from build123d import *

# Parameters (mm, degrees)
BOSS_EXTRUDE1_DEPTH                                 = 6.35
SKETCH2_W                                           = 6.35
SKETCH2_H                                           = 6.35
CUT_EXTRUDE1_DEPTH                                  = 7.35
F_8_0_199_DIAMETER_HOLE1_D                          = 5.0546
SKETCH5_W                                           = 6.35
SKETCH5_H                                           = 3.81
CUT_EXTRUDE2_DEPTH                                  = 7.35
CBORE_FOR_8_BINDING_HEAD_MACHINE_SCREW1_D           = 4.4958
CBORE_FOR_8_BINDING_HEAD_MACHINE_SCREW1_CBORE_D     = 9.525
CBORE_FOR_8_BINDING_HEAD_MACHINE_SCREW1_CBORE_DEPTH = 3.175


with BuildPart() as part:
    # Sketch1 → Boss-Extrude1 (new body)
    with BuildSketch(Plane(origin=(0, 0, 0), x_dir=(1, 0, 0), z_dir=(0, 1, 0))):
        Polygon((8.763, -10.331391255), (8.763, -15.411391255), (-1.905, -15.411391255), (-1.905, 7.448608745), (0, 7.448608745), (0, 192.868608745), (31.75, 192.868608745), (31.75, -10.331391255), align=None)
    extrude(amount=BOSS_EXTRUDE1_DEPTH)

    # Sketch2 → Cut-Extrude1 (cut, through all)
    with BuildSketch(Plane(origin=(0, 6.35, 0), x_dir=(1, 0, 0), z_dir=(0, 1, 0))):
        with Locations((3.175, 52.025608745)):
            Rectangle(SKETCH2_W, SKETCH2_H)
        with Locations((3.175, 100.285608745)):
            Rectangle(SKETCH2_W, SKETCH2_H)
        with Locations((3.175, 148.545608745)):
            Rectangle(SKETCH2_W, SKETCH2_H)
    extrude(amount=-CUT_EXTRUDE1_DEPTH, mode=Mode.SUBTRACT)

    # #8 (0.199) Diameter Hole1 (through all)
    with Locations(Plane(origin=(0, 6.35, 0), x_dir=(1, 0, 0), z_dir=(0, 1, 0))):
        with Locations((3.937, 2.368608745), (3.937, -10.331391255)):
            Hole(F_8_0_199_DIAMETER_HOLE1_D / 2)

    # Sketch5 → Cut-Extrude2 (cut, through all)
    with BuildSketch(Plane(origin=(0, 6.35, 0), x_dir=(1, 0, 0), z_dir=(0, 1, 0))):
        with Locations((3.175, -3.854391255)):
            Rectangle(SKETCH5_W, SKETCH5_H)
    extrude(amount=-CUT_EXTRUDE2_DEPTH, mode=Mode.SUBTRACT)

    # CBORE for #8 Binding Head Machine Screw1 (through all)
    with Locations(Plane(origin=(0, 6.35, 0), x_dir=(1, 0, 0), z_dir=(0, 1, 0))):
        with Locations((19.05, 173.818608745), (19.05, 142.068608745), (19.05, 15.068608745)):
            CounterBoreHole(CBORE_FOR_8_BINDING_HEAD_MACHINE_SCREW1_D / 2, CBORE_FOR_8_BINDING_HEAD_MACHINE_SCREW1_CBORE_D / 2, CBORE_FOR_8_BINDING_HEAD_MACHINE_SCREW1_CBORE_DEPTH)


solid = part.part
Read the model definition and answer for the solid it produces. Units are mm, in the model's axes. A direction names the side the tool comes from. Give positions to 0.01 mm unless a question says otherwise; leave off trailing zeros. Write each loop counter-clockwise with the first axis right and the second up, starting at its lowest first coordinate (ties: lowest second). Pieces come first, ordered by that corner, then holes. Notation, with made-up numbers: (-31.5, -20.75) - (12.5, -20.75) arc R14 ccw to (12.5, -10.75) - close; hole circle Ø7 at (-1.75, 69.25). An arc over 180 degrees is marked (long way). Use CSV: the item, a comma, the result in double quotes. Start each with the question number.
Item 1: For faces 4 (the flat face through (0, 3, -28)), 5 (the flat face through (3, 3, -48.851)), 6 (the cylindrical face through (15.54, 4.78, -18.29)), 7 (the flat face through (3, 3, 5.759)), determine the directions among +Z, -Z, +X, -X, +Y, -Y from which every point of the face is accessible in a straight line to the end or side of a thin tool.
Item 2: The mould has two halves that part along X. Classify faces 1 (the flat face through (20, 3.175, -17.3)), 2 (the flat face through (-1.905, 3, 4)), 3 (the flat face through (3, 3, -97.111)): pulls with the +X half, pulls with the -X half, needs draft (parallel to the pull), parting line crosses it, or undercut.
Item 3: Consider line 1 (Z direction, x = 19.05, y = 0.9); line 2 (Z direction, x = 19.5, y = 4); line 3 (X direction, y = 4, z = -2) (3 decimals). Determine where each line is inside the solid, lowest interval first.
Item 4: The part is cut by section A-A, the plane x = 19.05. Count the separate pieces of the cut face and the enclosed holes in it, and give its area (3 significant figures).
Item 5: The part is cut by section C-C, the plane z = -133.5. Give the vertices of the cut face in (x, y), and give its area (3 significant figures).
Item 6: Flat-ended cylindrical pins translate along their axes: P1, Ø5, axis at x = 18.5, z = -143.5, coming from the +Y side (3 decimals); P2, Ø8, axis at x = 24, z = -63, coming from the -Y side; P3, Ø3, axis at y = 3.5, z = -148, coming from the -X side; P4, Ø2.5, axis at y = 4, z = 13, coming from the +X side. Find the tip coordinate at first contact, or state that the pin passes through.
Taken from the geometry:
1,face 4,"-Z, -X, +Y, -Y"
1,face 5,"-X, +Y, -Y"
1,face 6,"+Y"
1,face 7,"+Y, -Y"
2,face 1,"undercut"
2,face 2,"pulls with the -X half"
2,face 3,"needs draft"
3,line 1,"-192.87 to -176.07, -171.57 to -144.32, -139.82 to -17.32, -12.82 to 10.33"
3,line 2,"-192.87 to -178.56, -169.08 to -146.81, -137.33 to -19.81, -10.33 to 10.33"
3,line 3,"-1.905 to 1.437, 6.437 to 31.75"
4,separate pieces,"4"
4,enclosed holes,"0"
4,area,"1,160 mm2"
5,outline,"(0, 0) - (31.75, 0) - (31.75, 6.35) - (0, 6.35) - close"
5,area,"202 mm2"
6,P1,"y = 3.175"
6,P2,"y = 0"
6,P3,"x = 6.35"
6,P4,"x = 8.76"
